```python
from build123d import *

# Parameters (mm, degrees)
F0_W     = 4.5
F0_H     = 150
F1_DEPTH = 7.3
F3_DEPTH = 10
F5_DEPTH = 15


with BuildPart() as f1:
    # F0 (on Top) → F1 (new body)
    with BuildSketch(Plane.XY):
        Rectangle(F0_W, F0_H)
    extrude(amount=F1_DEPTH)

    # F2 (on face) → F3 (join)
    with BuildSketch(Plane.XZ.offset(75)):
        Polygon((-2.25, 0.016098), (0, 0), (2.25, 0), (2.25, 7.3), (-2.25, 7.3), align=None)
        Polygon((4.999872, -0.035773), (5.107192, 14.963843), (-4.892552, 15.035389), (-4.999872, 0.035773), (-2.25, 0.016098), (-2.25, 7.3), (2.25, 7.3), (2.25, 0), (0, 0), align=None)
    extrude(amount=F3_DEPTH)

    # F4 (on face) → F5 (join)
    with BuildSketch(Plane(origin=(0.10732, 0, 14.999616), x_dir=(0.999974, 0, -0.007155), z_dir=(0.007155, 0, 0.999974))):
        Polygon((5, -85), (-5, -85), (-61.568542, -141.568542), (-56.568542, -146.568542), align=None)
    extrude(amount=-F5_DEPTH)


solid = f1.part
```
Build history of the part. All positions in model axes, mm. A direction names the side the tool comes from. Round coordinates to 2 decimals unless told otherwise and drop trailing zeros. Loops run counter-clockwise (first coordinate to the right, second up) from the corner with the lowest first, then second, coordinate; pieces in that order, holes last.
Item 1: Saw through at C-C (x = -38.5). List the corners of the cut face in (y, z), then the cut area to 3 significant figures.
Item 2: Drill centre lines: line 1 along X through (y, z) = (51, 1); line 2 along Y through (x, z) = (-8, 9.25); line 3 along X through (y, z) = (-81, 14.25). Where is each one in solid material? Low to high.
Item 3: Which spindle directions (+Z, -Z, +X, -X, +Y, -Y) get a long thin tool onto all of the face, cutting with end or side? Do faces 1 (the face through (0, 1, 7.3)), 2 (the face through (2.25, -1, 4)), 3 (the face through (-2.25, -1, 4)), 4 (the face through (0, 1, 0)). Say none if no direction does.
Item 4: Pin check, flat tips, straight feed: P1, Ø8, axis at y = -76.5, z = 4.5, coming from the -X side; P2, Ø3.5, axis at y = -9.5, z = 5, coming from the +X side; P3, Ø2, axis at x = -0.5, y = 3, coming from the -Z side. Stop position of each tip, or through.
Item 5: Saw through at B-B (y = -65.5). List the corners of the cut face in (x, z).
Worked answers:
1. outline: (-128.61, 15.28) - (-128.5, 0.28) - (-118.5, 0.28) - (-118.61, 15.28) - close
1. area: 150 mm2
2. line 1: x = -2.25 to 2.25
2. line 2: y = -98.07 to -88.07
2. line 3: x = -4.9 to 5.1
3. face 1: +Z, +X, -X, +Y
3. face 2: +Z, -Z, +X, +Y
3. face 3: +Z, -Z, -X, +Y
3. face 4: -Z, +X, -X, +Y, -Y
4. P1: stops at x = -5
4. P2: stops at x = 2.25
4. P3: stops at z = 0
5. outline: (-2.25, 0) - (2.25, 0) - (2.25, 7.3) - (-2.25, 7.3) - close
